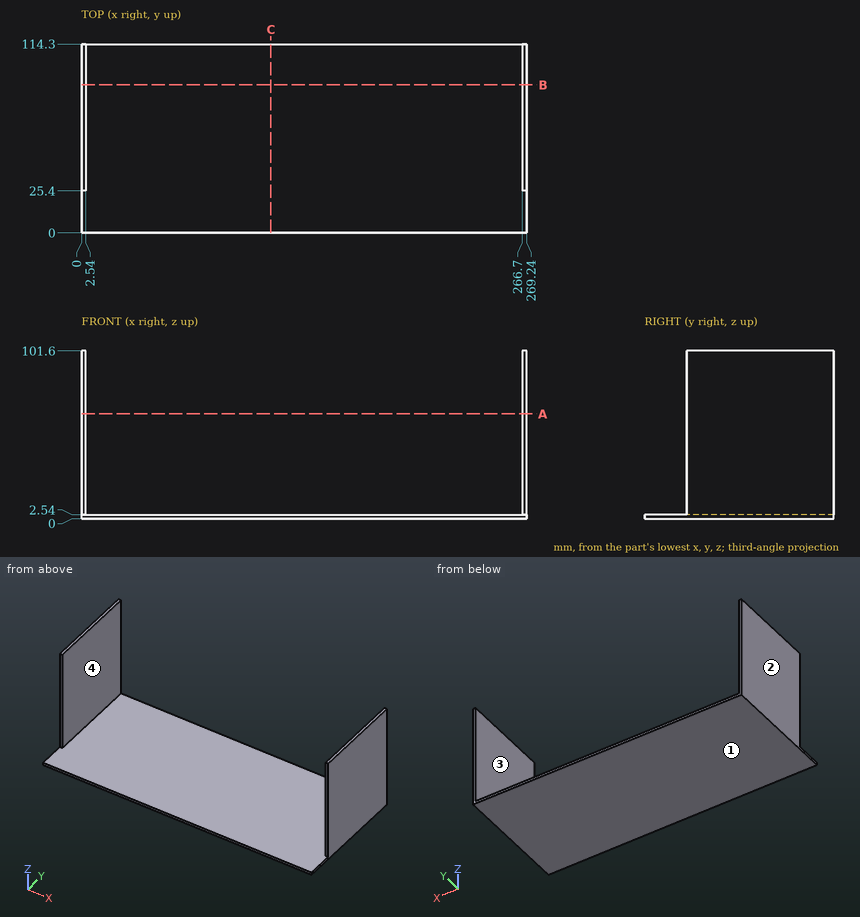
Part print with two shaded views. Sizes in mm from the minimum x, y, z corner. Give positions to 0.01 mm unless a question says otherwise; leave off trailing zeros. Order: outer loops, then holes, each group sorted by start corner. A loop starts at its lowest first (then second) coordinate and runs counter-clockwise, first axis right, second up. Notation, with made-up numbers: M -36,-33 L -24,-33 A25 cw -24,-3 Z; hole C -32.5,10.25 d6. An arc over 180 degrees is marked long. Put each result on its own line as item: value.
Item 1: Pull direction X, two halves, no side cores. Call the marked faces 1, 2, 3 and 4: +X half, -X half, draft (parallel to the pull), parting line (faces both ways), or undercut.
Results are:
face 1: draft
face 2: -X half
face 3: undercut
face 4: undercut
Item 2: Drop flat-ended pins along their axis: pin 1 Ø1.5 at (y, z) = (42.5, 45.5) entering from -X; pin 2 Ø2 at (x, z) = (268, 54) entering from -Y; pin 3 Ø2 at (x, y) = (96, 30.5) entering from +Z. Give the stop position or say it passes through.
Results are:
pin 1: x = 0
pin 2: y = 25.4
pin 3: z = 2.54
Item 3: Wall check: probe 1 along X at (y, z) = (89.5, 47); probe 2 along Z at (x, y) = (87.5, 48). Give the ranges that are in metal, low to high.
Results are:
probe 1: 0 to 2.54, 266.7 to 269.24
probe 2: 0 to 2.54
Item 4: Cut at A-A on z = 63.5. Write the cut outline in (x, y).
Results are:
outline: M 0,25.4 L 2.54,25.4 L 2.54,114.3 L 0,114.3 Z; M 266.7,25.4 L 269.24,25.4 L 269.24,114.3 L 266.7,114.3 Z
Item 5: Cut at C-C on x = 114.5. Write the cut outline in (y, z).
Results are:
outline: M 0,0 L 114.3,0 L 114.3,2.54 L 0,2.54 Z
Item 6: Cut at B-B on y = 89.5. Write the cut outline in (x, z).
Results are:
outline: M 0,0 L 269.24,0 L 269.24,101.6 L 266.7,101.6 L 266.7,2.54 L 2.54,2.54 L 2.54,101.6 L 0,101.6 Z
